Part model, mm, in its own coordinate system. Give positions to 0.01 mm unless a question says otherwise; leave off trailing zeros. Loops run counter-clockwise (first coordinate to the right, second up) from the corner with the lowest first, then second, coordinate; pieces in that order, holes last. Notation, with made-up numbers: M 74,38 L 129,38 A13 ccw 129,53 Z; hole C -39.75,42 d1. An arc over 180 degrees is marked long. Answer in a Markdown table with one row per item.
from build123d import *

# Parameters (mm, degrees)
CUT_EXTRUDE1_DEPTH   = 10
FILLET1_R            = 1
M2_CLEARANCE_HOLE2_D = 2.4
CIRPATTERN1_COUNT    = 4


with BuildPart() as part:
    # Sketch2 → Revolve1 (revolve)
    with BuildSketch(Plane.XY):
        Polygon((0, 0), (0, 8.5), (-6.2, 8.5), (-6.2, 1), (-10, 1), (-10, 0), align=None)
    revolve(axis=Axis((0, 0, 0), (0, 1, 0)))

    # Sketch3 → Cut-Extrude1 (cut)
    with BuildSketch(Plane(origin=(0, 8.5, 0), x_dir=(1, 0, 0), z_dir=(0, 1, 0))):
        with BuildLine():
            Line((-2.6, 2.112463017), (-2.6, -2.112463017))
            ThreePointArc((-2.6, -2.112463017), (3.35, 0), (-2.6, 2.112463017))
        make_face()
    extrude(amount=-CUT_EXTRUDE1_DEPTH, mode=Mode.SUBTRACT)

    # Fillet1
    fillet1_edges = [part.edges().sort_by_distance(p)[0] for p in [
        (6.2, 1, 0),
        (6.2, 8.5, 0),
    ]]
    fillet(fillet1_edges, radius=FILLET1_R)

    # M2 Clearance Hole2 (through all)
    with Locations(Plane(origin=(0, 0, 0), x_dir=(-1, 0, 0), z_dir=(0, -1, 0))):
        with Locations((8, 0)):
            m2_clearance_hole2 = Hole(M2_CLEARANCE_HOLE2_D / 2)

    # CirPattern1: M2 Clearance Hole2 ×4 about axis
    cirpattern1_axis = Axis((0, 0, 0), (0, 1, 0))
    for i in range(1, CIRPATTERN1_COUNT):
        add(m2_clearance_hole2.rotate(cirpattern1_axis, i * 360 / CIRPATTERN1_COUNT), mode=Mode.SUBTRACT)


solid = part.part
(1) Saw through at D-D (y = 0.75). Write the cut outline in (x, z), plus the area to 3 significant figures.
Recorded:
| item | result |
|---|---|
| outline | C 0,0 d20; hole C -8,0 d2.4; hole M -2.6,-2.11 A3.35 ccw long -2.6,2.11 Z; hole C 0,-8 d2.4; hole C 0,8 d2.4; hole C 8,0 d2.4 |
| area | 263 mm^2 |
(2) Pin check, flat tips, straight feed: pin 1 Ø3 at (x, z) = (8, 0) entering from +Y; pin 2 Ø3.5 at (y, z) = (3.5, 0) entering from +X; pin 3 Ø1.5 at (x, y) = (5, 7) entering from -Z. Stop position of each tip, or through.
Recorded:
| item | result |
|---|---|
| pin 1 | stops at y = 1.29 |
| pin 2 | stops at x = 6.23 |
| pin 3 | stops at z = -4.51 |
(3) Saw through at A-A (x = 0). Write the cut outline in (y, z).
Recorded:
| item | result |
|---|---|
| outline | M 0,-10 L 1,-10 L 1,-9.2 L 0,-9.2 Z; M 0,-6.8 L 1.08,-6.8 A1 cw 2,-6.2 L 7.5,-6.2 A1 ccw 8.5,-5.2 L 8.5,-3.35 L 0,-3.35 Z; M 0,3.35 L 8.5,3.35 L 8.5,5.2 A1 ccw 7.5,6.2 L 2,6.2 A1 cw 1.08,6.8 L 0,6.8 Z; M 0,9.2 L 1,9.2 L 1,10 L 0,10 Z |
(4) Drill centre lines: line 1 along Z through (x, y) = (-0.75, 3); line 2 along X through (y, z) = (5.75, 0.25); line 3 along X through (y, z) = (2.25, 1). Where is each one in solid material? Low to high.
Recorded:
| item | result |
|---|---|
| line 1 | z = -6.15 to -3.26, 3.26 to 6.15 |
| line 2 | x = -6.19 to -2.6, 3.34 to 6.19 |
| line 3 | x = -6.12 to -2.6, 3.2 to 6.12 |
(5) Saw through at B-B (z = 8). Write the cut outline in (x, y), plus the area to 3 significant figures.
Recorded:
| item | result |
|---|---|
| outline | M -6,0 L -1.2,0 L -1.2,1 L -6,1 Z; M 1.2,0 L 6,0 L 6,1 L 1.2,1 Z |
| area | 9.60 mm^2 |
(6) Saw through at C-C (x = 8). Write the cut outline in (y, z), plus the area to 3 significant figures.
Recorded:
| item | result |
|---|---|
| outline | M 0,-6 L 1,-6 L 1,-1.2 L 0,-1.2 Z; M 0,1.2 L 1,1.2 L 1,6 L 0,6 Z |
| area | 9.60 mm^2 |
(7) Pull direction Z, two halves, no side cores. Call faces 1 (the face through (-2.6, 4, 0)), 2 (the face through (5.9, 1, -4.4)), 3 (the face through (-2.86, 4.71, -5.5)): +Z half, -Z half, draft (parallel to the pull), parting line (faces both ways), or undercut.
Recorded:
| item | result |
|---|---|
| face 1 | undercut |
| face 2 | draft |
| face 3 | parting line |
